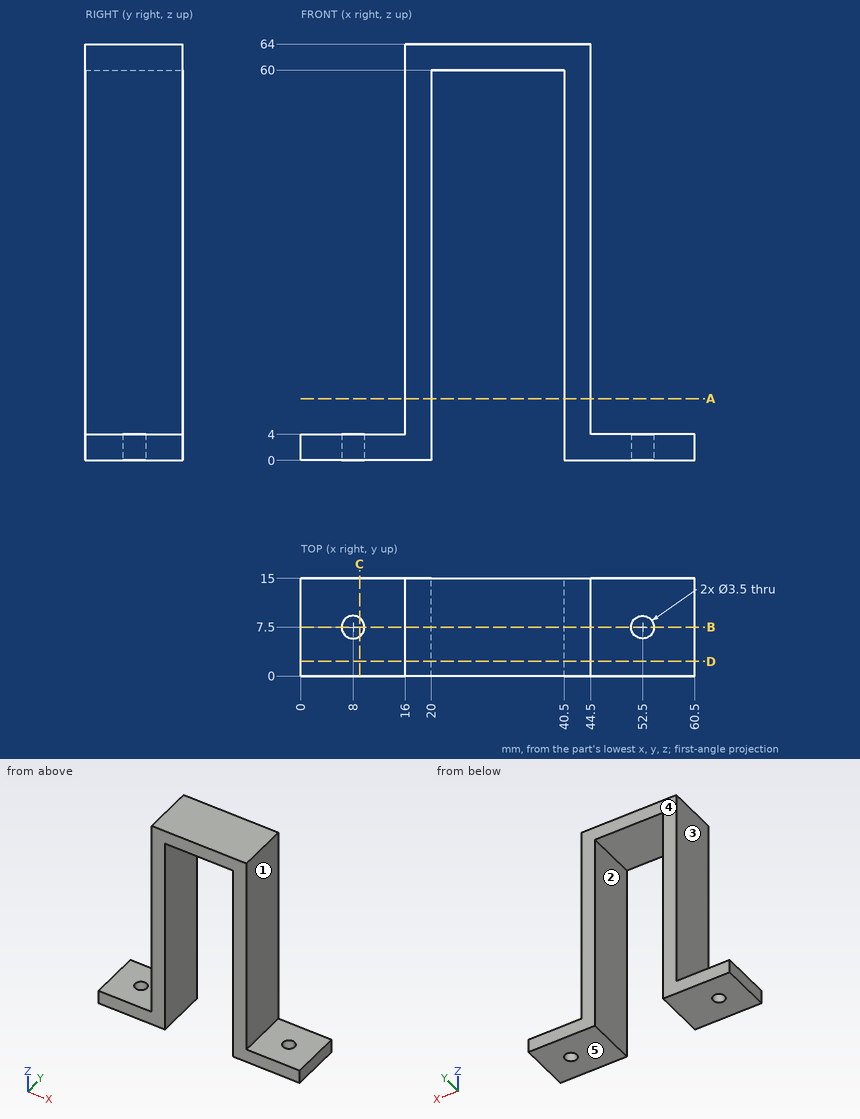
Input: dimensioned drawing with shaded views. Units: mm. Origin: part minimum x, y, z. A direction names the side the tool comes from. Coordinates: 2 decimals unless noted, no trailing zeros. Order: outer loops, then holes, each group sorted by start corner. A loop starts at its lowest first (then second) coordinate and runs counter-clockwise, first axis right, second up. Notation, with made-up numbers: M -13,11.5 L 19,11.5 A6 cw 19,16.5 Z; hole C 29.5,-8 d8. An arc over 180 degrees is marked long. Write each question's results on one line, items separated by ' | '. Start each with the question number.
Item 1: Cut plane D-D (y = 2.25). Return loops of the section in (x, z).
Item 2: Set-up query: the marked faces 1, 2, 3, 4 and 5. Return all of +Z, -Z, +X, -X, +Y, -Y with unobstructed straight access to the full face (end or side cutting, diameter ignored); none if empty.
Item 3: Cut plane B-B (y = 7.5). Return loops of the section in (x, z), and give its area (3 significant figures).
Item 4: Cut plane C-C (x = 9). Return loops of the section in (y, z).
Item 5: First-contact query: pin 1 Ø3 at (y, z) = (9, 41.5) entering from +X; pin 2 Ø5 at (x, y) = (29.5, 6) entering from -Z; pin 3 Ø4 at (x, y) = (52.5, 7.5) entering from -Z; pin 4 Ø3 at (x, y) = (8, 7.5) entering from -Z. Flat tips, straight axial feed; report the tip coordinate or a pass-through.
Item 6: Line query: probe 1 along X at (y, z) = (7.5, 1.25); probe 2 along X at (y, z) = (11.25, 11.5); probe 3 along Z at (x, y) = (56, 3). Output: solid intervals per line, ascending.
Item 7: Cut plane A-A (z = 9.5). Return loops of the section in (x, y), and give its area (3 significant figures).
Checked values:
1) outline: M 0,0 L 20,0 L 20,60 L 40.5,60 L 40.5,0 L 60.5,0 L 60.5,4 L 44.5,4 L 44.5,64 L 16,64 L 16,4 L 0,4 Z
2) face 1: +Z, +X, +Y, -Y | face 2: -Z, +Y, -Y | face 3: +Z, -X, +Y, -Y | face 4: +Z, -Z, +X, -X, +Y | face 5: -Z, +X, -X, +Y, -Y
3) outline: M 0,0 L 6.25,0 L 6.25,4 L 0,4 Z; M 9.75,0 L 20,0 L 20,60 L 40.5,60 L 40.5,0 L 50.75,0 L 50.75,4 L 44.5,4 L 44.5,64 L 16,64 L 16,4 L 9.75,4 Z; M 54.25,0 L 60.5,0 L 60.5,4 L 54.25,4 Z | area: 694 mm2
4) outline: M 0,0 L 6.06,0 L 6.06,4 L 0,4 Z; M 8.94,0 L 15,0 L 15,4 L 8.94,4 Z
5) pin 1: stops at x = 44.5 | pin 2: stops at z = 60 | pin 3: stops at z = 0 | pin 4: passes through
6) probe 1: x = 0 to 6.25, 9.75 to 20, 40.5 to 50.75, 54.25 to 60.5 | probe 2: x = 16 to 20, 40.5 to 44.5 | probe 3: z = 0 to 4
7) outline: M 16,0 L 20,0 L 20,15 L 16,15 Z; M 40.5,0 L 44.5,0 L 44.5,15 L 40.5,15 Z | area: 120 mm2
